Drawing for the job (mm, zero at the part's lowest x, y, z). Coordinates: 2 decimals unless noted, no trailing zeros. Write each loop counter-clockwise with the first axis right and the second up, starting at its lowest first coordinate (ties: lowest second). Pieces come first, ordered by that corner, then holes. Notation, with made-up numbers: (-3, 48) -> (39, 48) arc R30 cw to (39, 79) -> close; hole circle Ø1 at (80.25, -15.5). An arc over 180 degrees is marked (long way). Write item = value, one per line. Start each with the question number.
Q1. Band-saw the part on D-D, the plane y = 1.75. List the corners of the cut face in (x, z).
Q2. Probe line 1 (X direction, y = 23, z = 2.6); line 2 (Y direction, x = 15.5, z = 2.6); line 3 (X direction, y = 9.75, z = 2.3). List the from-to ranges inside material, lowest first.
Q3. Band-saw the part on C-C, the plane x = 7. List the corners of the cut face in (y, z).
Q4. Band-saw the part on B-B, the plane z = 0.9. List the corners of the cut face in (x, y).
Q5. Band-saw the part on A-A, the plane y = 22.5. List the corners of the cut face in (x, z).
Q6. Pin check, flat tips, straight feed: P1, Ø1, axis at x = 9, z = 2, coming from the +Y side; P2, Ø1, axis at y = 8, z = 1.5, coming from the -X side; P3, Ø1.5, axis at y = 1.5, z = 2, coming from the +X side. Stop position of each tip, or through.
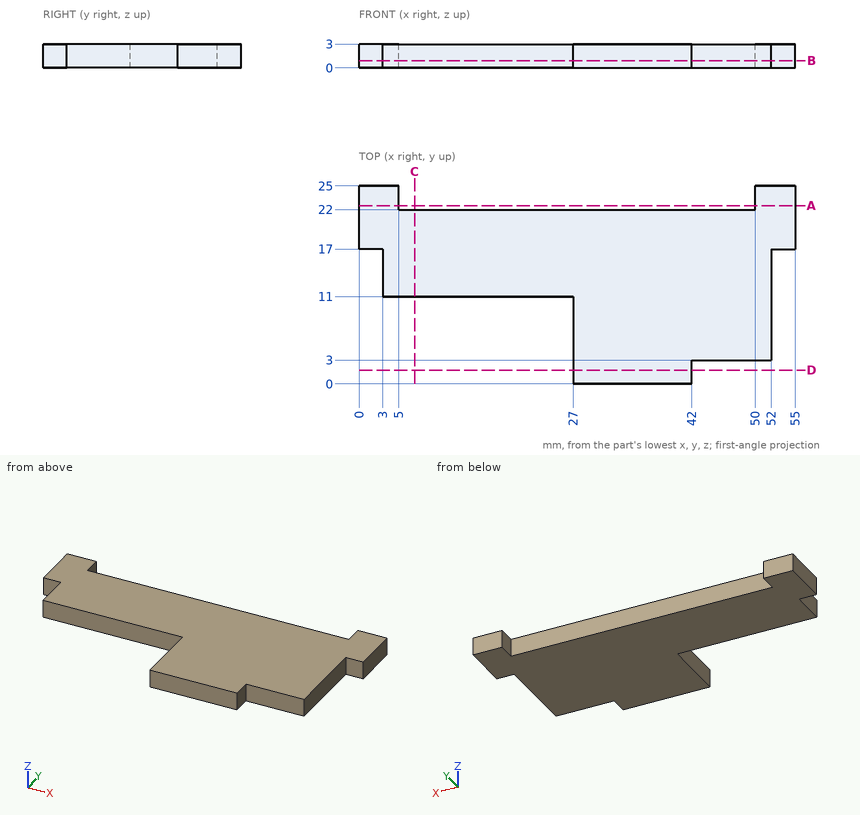
Ans:
q1.outline = (27, 0) -> (42, 0) -> (42, 3) -> (27, 3) -> close
q2.line_1 = 0 to 5, 50 to 55
q2.line_2 = 11 to 22
q2.line_3 = 27 to 52
q3.outline = (11, 0) -> (22, 0) -> (22, 3) -> (11, 3) -> close
q4.outline = (0, 17) -> (3, 17) -> (3, 11) -> (27, 11) -> (27, 0) -> (42, 0) -> (42, 3) -> (52, 3) -> (52, 17) -> (55, 17) -> (55, 25) -> (50, 25) -> (50, 22) -> (5, 22) -> (5, 25) -> (0, 25) -> close
q5.outline = (0, 0) -> (5, 0) -> (5, 3) -> (0, 3) -> close; (50, 0) -> (55, 0) -> (55, 3) -> (50, 3) -> close
q6.P1 = 22
q6.P2 = 27
q6.P3 = 42
